from build123d import *

# Parameters (mm, degrees)
F0_W      = 76.2
F0_H      = 12.7
F1_DEPTH  = 3.175
F2_W      = 6.35
F2_H      = 12.7
F2_W_2    = 12.7
F3_DEPTH  = 8.255
F4_W      = 6.35
F4_H      = 4.191
F4_W_2    = 12.7
F5_DEPTH  = 3.175
F7_DEPTH  = 6.35
F9_DEPTH  = 12.7
F11_DEPTH = 12.7
F13_DEPTH = 12.7
F15_DEPTH = 6.35
F17_DEPTH = 12.7
F18_R     = 3.175


with BuildPart() as f1:
    # F0 (on Top) → F1 (new body)
    with BuildSketch(Plane.XY):
        with Locations((-12.1522513986, 0.3075693393)):
            Rectangle(F0_W, F0_H)
    extrude(amount=F1_DEPTH)

    # F2 (on face) → F3 (join)
    with BuildSketch(Plane.XY.offset(3.175)):
        with Locations((-47.0772513986, 0.3075693393)):
            Rectangle(F2_W, F2_H)
        with Locations((-31.2022513986, 0.3075693393)):
            Rectangle(F2_W_2, F2_H)
        with Locations((-12.1522513986, 0.3075693393)):
            Rectangle(F2_W_2, F2_H)
        with Locations((6.8977486014, 0.3075693393)):
            Rectangle(F2_W_2, F2_H)
        with Locations((22.7727486014, 0.3075693393)):
            Rectangle(F2_W, F2_H)
    extrude(amount=F3_DEPTH)

    # F4 (on face) → F5 (join)
    with BuildSketch(Plane.XZ.offset(6.0424306607)):
        with Locations((-47.0772513986, 9.3345)):
            Rectangle(F4_W, F4_H)
        with Locations((-31.2022513986, 9.3345)):
            Rectangle(F4_W_2, F4_H)
        with Locations((-12.1522513986, 9.3345)):
            Rectangle(F4_W_2, F4_H)
        with Locations((6.8977486014, 9.3345)):
            Rectangle(F4_W_2, F4_H)
        with Locations((22.7727486014, 9.3345)):
            Rectangle(F4_W, F4_H)
    extrude(amount=F5_DEPTH)

    # F6 (on face) → F7 (join)
    with BuildSketch(Plane.YZ.offset(25.9477486014)):
        with BuildLine():
            Line((-6.0424306607, 7.239), (-7.7569306607, 7.239))
            ThreePointArc((-7.7569306607, 7.239), (-6.5445960844, 6.7368345763), (-6.0424306607, 5.5245))
            Line((-6.0424306607, 5.5245), (-6.0424306607, 7.239))
        make_face()
    extrude(amount=-F7_DEPTH)

    # F8 (on face) → F9 (join)
    with BuildSketch(Plane.YZ.offset(13.2477486014)):
        with BuildLine():
            Line((-6.0424306607, 7.239), (-7.7569306607, 7.239))
            ThreePointArc((-7.7569306607, 7.239), (-6.5445960844, 6.7368345763), (-6.0424306607, 5.5245))
            Line((-6.0424306607, 5.5245), (-6.0424306607, 7.239))
        make_face()
    extrude(amount=-F9_DEPTH)

    # F10 (on face) → F11 (join)
    with BuildSketch(Plane.YZ.offset(-5.8022513986)):
        with BuildLine():
            Line((-6.0424306607, 7.239), (-7.7569306607, 7.239))
            ThreePointArc((-7.7569306607, 7.239), (-6.5445960844, 6.7368345763), (-6.0424306607, 5.5245))
            Line((-6.0424306607, 5.5245), (-6.0424306607, 7.239))
        make_face()
    extrude(amount=-F11_DEPTH)

    # F12 (on face) → F13 (join)
    with BuildSketch(Plane.YZ.offset(-24.8522513986)):
        with BuildLine():
            Line((-6.0424306607, 7.239), (-7.7569306607, 7.239))
            ThreePointArc((-7.7569306607, 7.239), (-6.5445960844, 6.7368345763), (-6.0424306607, 5.5245))
            Line((-6.0424306607, 5.5245), (-6.0424306607, 7.239))
        make_face()
    extrude(amount=-F13_DEPTH)

    # F14 (on face) → F15 (join)
    with BuildSketch(Plane.YZ.offset(-43.9022513986)):
        with BuildLine():
            Line((-6.0424306607, 7.239), (-7.7569306607, 7.239))
            ThreePointArc((-7.7569306607, 7.239), (-6.5445960844, 6.7368345763), (-6.0424306607, 5.5245))
            Line((-6.0424306607, 5.5245), (-6.0424306607, 7.239))
        make_face()
    extrude(amount=-F15_DEPTH)

    # F16 (on face) → F17 (join)
    with BuildSketch(Plane.XZ.offset(6.0424306607)):
        with BuildLine():
            ThreePointArc((-40.7272513986, 3.175), (-42.9723154288, 4.1049359697), (-43.9022513986, 6.35))
            Line((-43.9022513986, 6.35), (-43.9022513986, 5.5245))
            Line((-43.9022513986, 5.5245), (-43.9022513986, 3.175))
            Line((-43.9022513986, 3.175), (-40.7272513986, 3.175))
        make_face()
        with BuildLine():
            ThreePointArc((-37.5522513986, 6.35), (-38.4821873683, 4.1049359697), (-40.7272513986, 3.175))
            Line((-40.7272513986, 3.175), (-37.5522513986, 3.175))
            Line((-37.5522513986, 3.175), (-37.5522513986, 5.5245))
            Line((-37.5522513986, 5.5245), (-37.5522513986, 6.35))
        make_face()
        with BuildLine():
            Line((-24.8522513986, 6.35), (-24.8522513986, 5.5245))
            Line((-24.8522513986, 5.5245), (-24.8522513986, 3.175))
            Line((-24.8522513986, 3.175), (-21.6772513986, 3.175))
            ThreePointArc((-21.6772513986, 3.175), (-23.9223154288, 4.1049359697), (-24.8522513986, 6.35))
        make_face()
        with BuildLine():
            ThreePointArc((-18.5022513986, 6.35), (-19.4321873683, 4.1049359697), (-21.6772513986, 3.175))
            Line((-21.6772513986, 3.175), (-18.5022513986, 3.175))
            Line((-18.5022513986, 3.175), (-18.5022513986, 5.5245))
            Line((-18.5022513986, 5.5245), (-18.5022513986, 6.35))
        make_face()
        with BuildLine():
            Line((-5.8022513986, 6.35), (-5.8022513986, 5.5245))
            Line((-5.8022513986, 5.5245), (-5.8022513986, 3.175))
            Line((-5.8022513986, 3.175), (-2.6272513986, 3.175))
            ThreePointArc((-2.6272513986, 3.175), (-4.8723154288, 4.1049359697), (-5.8022513986, 6.35))
        make_face()
        with BuildLine():
            Line((0.5477486014, 3.175), (0.5477486014, 5.5245))
            Line((0.5477486014, 5.5245), (0.5477486014, 6.35))
            ThreePointArc((0.5477486014, 6.35), (-0.3821873683, 4.1049359697), (-2.6272513986, 3.175))
            Line((-2.6272513986, 3.175), (0.5477486014, 3.175))
        make_face()
        with BuildLine():
            Line((13.2477486014, 3.175), (16.4227486014, 3.175))
            ThreePointArc((16.4227486014, 3.175), (14.1776845712, 4.1049359697), (13.2477486014, 6.35))
            Line((13.2477486014, 6.35), (13.2477486014, 5.5245))
            Line((13.2477486014, 5.5245), (13.2477486014, 3.175))
        make_face()
        with BuildLine():
            Line((19.5977486014, 3.175), (19.5977486014, 5.5245))
            Line((19.5977486014, 5.5245), (19.5977486014, 6.35))
            ThreePointArc((19.5977486014, 6.35), (18.6678126317, 4.1049359697), (16.4227486014, 3.175))
            Line((16.4227486014, 3.175), (19.5977486014, 3.175))
        make_face()
    extrude(amount=-F17_DEPTH)

    # F18
    f18_edges = [f1.edges().sort_by_distance(p)[0] for p in [
        (22.772749, 6.657569, 11.43),
        (6.897749, 6.657569, 11.43),
        (-12.152251, 6.657569, 11.43),
        (-31.202251, 6.657569, 11.43),
        (-47.077251, 6.657569, 11.43),
        (-47.077251, -9.217431, 11.43),
        (-31.202251, -9.217431, 11.43),
        (-12.152251, -9.217431, 11.43),
        (6.897749, -9.217431, 11.43),
        (22.772749, -9.217431, 11.43),
        (-50.252251, 6.657569, 5.715),
        (25.947749, 6.657569, 5.715),
    ]]
    fillet(f18_edges, radius=F18_R)


solid = f1.part
Can you work these out from the model? Positions are in its coordinate system, mm. A direction names the side the tool comes from. Give positions to 0.01 mm unless a question says otherwise; leave off trailing zeros. Loops run counter-clockwise (first coordinate to the right, second up) from the corner with the lowest first, then second, coordinate; pieces in that order, holes last. Notation, with made-up numbers: M 89.5,-37 L 131.5,-37 A20 cw 131.5,-20 Z; hole C -7.5,15 d4. An arc over 180 degrees is marked long. One line per item, written item: value. Start each with the question number.
1) If we section it at B-B, the plane y = -4.5: Write out the boundary of the cut face in (x, z) (3 decimals), and give its area (3 significant figures).
2) If we section it at C-C, the plane z = 10: Write out the boundary of the cut face in (x, y) (3 decimals), and give its area (3 significant figures).
3) On a 3-axis mill with a long thin cutter (end or side, diameter ignored), from which of +Z, -Z, +X, -X, +Y, -Y can I reach the whole of each face in a straight line? I mean faces 1 (the face through (-12, -8, 7.239)), 2 (the face through (-5.802, -1, 9)), 3 (the face through (-13, 6.658, 3)). Say none if no direction works.
4) I'm going to push flat-ended pins straight in: pin 1 (1.6 mm diameter, centred on x = -47.5, y = -8, fed in from -Z); pin 2 (1.2 mm diameter, centred on x = 24, y = -8.5, fed in from -Z); pin 3 (2 mm diameter, centred on x = -40, y = -6, fed in from +Z). Where does each tip first touch, or does it pass through?
5) If we section it at D-D, the plane z = 1: Write out the boundary of the cut face in (x, y) (3 decimals).
6) If I drill on line 1 (X direction, y = 3.5, z = 9); line 2 (Y direction, x = -12.5, z = 8.5); line 3 (Y direction, x = -37.5, z = 2.75), over which ranges is the centre line in solid material (lowest first)? Write a range as [from, to].
7) Thinking about a two-plate mould opening in X: for faces 4 (the face through (-47.03, -8.31, 10.48)), 5 (the face through (24.993, 5.752, 5.635)), 6 (the face through (-18.502, -1, 9)), which applies, +X half, -X half, draft (parallel to the pull), parting line (faces both ways), or undercut?
Completed:
1. outline: M -50.252,0 L 25.948,0 L 25.948,11.43 L 19.598,11.43 L 19.598,6.35 A3.175 cw 13.248,6.35 L 13.248,11.43 L 0.548,11.43 L 0.548,6.35 A3.175 cw -5.802,6.35 L -5.802,11.43 L -18.502,11.43 L -18.502,6.35 A3.175 cw -24.852,6.35 L -24.852,11.43 L -37.552,11.43 L -37.552,6.35 A3.175 cw -43.902,6.35 L -43.902,11.43 L -50.252,11.43 Z
1. area: 679 mm^2
2. outline: M -50.252,-8.695 L -43.902,-8.695 L -43.902,6.135 L -48.822,6.135 A3.175 ccw -50.252,3.483 Z; M -37.552,-8.695 L -24.852,-8.695 L -24.852,6.135 L -37.552,6.135 Z; M -18.502,-8.695 L -5.802,-8.695 L -5.802,6.135 L -18.502,6.135 Z; M 0.548,-8.695 L 13.248,-8.695 L 13.248,6.135 L 0.548,6.135 Z; M 19.598,-8.695 L 25.948,-8.695 L 25.948,3.483 A3.175 ccw 24.518,6.135 L 19.598,6.135 Z
2. area: 751 mm^2
3. face 1: -Z, +X, -X, -Y
3. face 2: +Z, +Y, -Y
3. face 3: +Z, -Z, +X, -X, +Y
4. pin 1: stops at z = 7.15
4. pin 2: stops at z = 7.24
4. pin 3: stops at z = 3.69
5. outline: M -50.252,-6.042 L 25.948,-6.042 L 25.948,3.483 A3.175 ccw 22.773,6.658 L -47.077,6.658 A3.175 ccw -50.252,3.483 Z
6. line 1: x = [-50.25, -43.9], [-37.55, -24.85], [-18.5, -5.8], [0.55, 13.25], [19.6, 25.95]
6. line 2: y = [-9.21, 6.65]
6. line 3: y = [-6.04, 6.66]
7. face 4: draft
7. face 5: +X half
7. face 6: undercut
